```python
from build123d import *

# Parameters (mm, degrees)
SKETCH1_W           = 30
SKETCH1_H           = 27
SKETCH1_W_2         = 26
SKETCH1_H_2         = 23
BOSS_EXTRUDE1_DEPTH = 43
SKETCH3_W           = 30
SKETCH3_H           = 15
BOSS_EXTRUDE2_DEPTH = 2
SKETCH5_W           = 15
SKETCH5_H           = 2
SKETCH5_W_2         = 5
BOSS_EXTRUDE3_DEPTH = 10
BOSS_EXTRUDE4_DEPTH = 5
SKETCH7_W           = 5
SKETCH7_H           = 2
CUT_EXTRUDE1_DEPTH  = 5
FILLET3_R           = 0.5
SKETCH8_W           = 26
SKETCH8_H           = 10
CUT_EXTRUDE2_DEPTH  = 10


with BuildPart() as part:
    # Sketch1 → Boss-Extrude1 (new body)
    with BuildSketch(Plane.XY):
        Rectangle(SKETCH1_W, SKETCH1_H)
        Rectangle(SKETCH1_W_2, SKETCH1_H_2, mode=Mode.SUBTRACT)
    extrude(amount=BOSS_EXTRUDE1_DEPTH)

    # Sketch3 → Boss-Extrude2 (add)
    with BuildSketch(Plane(origin=(0, 0, 0), x_dir=(-1, 0, 0), z_dir=(0, 0, -1))):
        with Locations((0, 6)):
            Rectangle(SKETCH3_W, SKETCH3_H)
    extrude(amount=-BOSS_EXTRUDE2_DEPTH)

    # Sketch5 → Boss-Extrude3 (add)
    with BuildSketch(Plane(origin=(0, 0, 0), x_dir=(-1, 0, 0), z_dir=(0, 0, -1))):
        with Locations((0, -0.5)):
            Rectangle(SKETCH5_W, SKETCH5_H)
        with Locations((0, -12.5)):
            Rectangle(SKETCH5_W_2, SKETCH5_H)
    extrude(amount=BOSS_EXTRUDE3_DEPTH)

    # Sketch6 → Boss-Extrude4 (add)
    with BuildSketch(Plane.ZY.offset(2.5)):
        Polygon((-5, -13.5), (-3, -15.5), (-3, -13.5), align=None)
    extrude(amount=-BOSS_EXTRUDE4_DEPTH)

    # Sketch7 → Cut-Extrude1 (cut)
    with BuildSketch(Plane(origin=(0, 0, -10), x_dir=(-1, 0, 0), z_dir=(0, 0, -1))):
        with Locations((0, -12.5)):
            Rectangle(SKETCH7_W, SKETCH7_H)
    extrude(amount=-CUT_EXTRUDE1_DEPTH, mode=Mode.SUBTRACT)

    # Fillet3
    fillet3_edges = [part.edges().sort_by_distance(p)[0] for p in [
        (0, -13.5, -5),
        (0, -15.5, -3),
        (0, -11.5, -5),
    ]]
    fillet(fillet3_edges, radius=FILLET3_R)

    # Sketch8 → Cut-Extrude2 (cut)
    with BuildSketch(Plane(origin=(0, 13.5, 0), x_dir=(1, 0, 0), z_dir=(0, 1, 0))):
        with Locations((0, -7)):
            Rectangle(SKETCH8_W, SKETCH8_H)
    extrude(amount=-CUT_EXTRUDE2_DEPTH, mode=Mode.SUBTRACT)


solid = part.part
```
Build history of the part. All positions in model axes, mm. A direction names the side the tool comes from. Coordinates: 2 decimals unless noted, no trailing zeros. Write each loop counter-clockwise with the first axis right and the second up, starting at its lowest first coordinate (ties: lowest second). Pieces come first, ordered by that corner, then holes.
1. Band-saw the part on C-C, the plane z = 26.5. Give the cut face in (x, y), and give its area (3 significant figures).
Answer block:
outline: (-15, -13.5) - (15, -13.5) - (15, 13.5) - (-15, 13.5) - close; hole (-13, -11.5) - (13, -11.5) - (13, 11.5) - (-13, 11.5) - close
area: 212 mm2
2. Band-saw the part on D-D, the plane x = 4.25. Give the cut face in (y, z).
Answer block:
outline: (-13.5, 0) - (-11.5, 0) - (-11.5, 43) - (-13.5, 43) - close; (-1.5, -10) - (0.5, -10) - (0.5, 0) - (13.5, 0) - (13.5, 2) - (-1.5, 2) - close; (11.5, 12) - (13.5, 12) - (13.5, 43) - (11.5, 43) - close
3. Drill centre lines: probe 1 along X at (y, z) = (7.75, 12.5); probe 2 along Y at (x, z) = (-0.25, 32); probe 3 along Y at (x, z) = (0.5, -2). Where is each one in solid material? Low to high.
Answer block:
probe 1: x = -15 to -13, 13 to 15
probe 2: y = -13.5 to -11.5, 11.5 to 13.5
probe 3: y = -13.5 to -11.5, -1.5 to 0.5
4. Band-saw the part on A-A, the plane x = 9. Give the cut face in (y, z), and give its area (3 significant figures).
Answer block:
outline: (-13.5, 0) - (-11.5, 0) - (-11.5, 43) - (-13.5, 43) - close; (-1.5, 0) - (13.5, 0) - (13.5, 2) - (-1.5, 2) - close; (11.5, 12) - (13.5, 12) - (13.5, 43) - (11.5, 43) - close
area: 178 mm2
5. Drop flat-ended pins along their axis: pin 1 (3 mm diameter, centred on y = 1.5, z = -3.5, fed in from -X); pin 2 (2.5 mm diameter, centred on y = -14, z = -3.5, fed in from -X); pin 3 (2 mm diameter, centred on x = 0, y = 12, fed in from -Z). Give the stop position or say it passes through.
Answer block:
pin 1: stops at x = -7.5
pin 2: stops at x = -2.5
pin 3: stops at z = 0
6. Band-saw the part on B-B, the plane y = -9.5. Give the cut face in (x, z).
Answer block:
outline: (-15, 0) - (-13, 0) - (-13, 43) - (-15, 43) - close; (13, 0) - (15, 0) - (15, 43) - (13, 43) - close
7. Pull direction X, two halves, no side cores. Call faces 6 (the flat face through (0, -1.5, -4)), 7 (the flat face through (0, 13.5, 26)), 8 (the flat face through (7.5, -1, -5)): released by +X, released by -X, zero draft, split by the parting line, or undercut.
Answer block:
face 6: undercut
face 7: zero draft
face 8: released by +X
8. 3-axis set-ups, long thin cutter, end or side, ignore diameter. For faces 1 (the flat face through (0, 0.5, -5)), 2 (the flat face through (2.5, -13, -2)), 3 (the flat face through (-2.5, -13, -2)), 4 (the flat face through (0, 11.5, 27)), 5 (the flat face through (0, -13.5, 20)): which of +Z, -Z, +X, -X, +Y, -Y reach the whole face in a straight line?
Answer block:
face 1: -Z, +X, -X, +Y
face 2: -Z, +X, -Y
face 3: -Z, -X, -Y
face 4: +Z
face 5: +Z, +X, -X, -Y
